from build123d import *

# Parameters (mm, degrees)
SKETCH1_W          = 190.5
SKETCH1_H          = 114.3
SKETCH1_R          = 2.413
SKETCH1_W_2        = 127
SKETCH1_H_2        = 82.55
BASE_FLANGE1_DEPTH = 2.38125
FILLET1_R          = 6.35
SKETCH2_W          = 36.53028
SKETCH2_H          = 15.875
CUT_EXTRUDE1_DEPTH = 2.54
FILLET2_R          = 6.35


# Sheet-metal steps are written as plain solids
with BuildPart() as part:
    # Sketch1 → Base-Flange1 (new body)
    with BuildSketch(Plane(origin=(0, 0, 0), x_dir=(1, 0, 0), z_dir=(0, 1, 0))):
        Rectangle(SKETCH1_W, SKETCH1_H)
        with Locations(Location((-76.2, -51.59375, 0), (0, 0, 270))):
            Circle(SKETCH1_R, mode=Mode.SUBTRACT)
        with Locations(Location((-50.8, -51.59375, 0), (0, 0, 270))):
            Circle(SKETCH1_R, mode=Mode.SUBTRACT)
        with Locations(Location((-25.4, -51.59375, 0), (0, 0, 270))):
            Circle(SKETCH1_R, mode=Mode.SUBTRACT)
        with Locations(Location((0, -51.59375, 0), (0, 0, 270))):
            Circle(SKETCH1_R, mode=Mode.SUBTRACT)
        with Locations(Location((25.4, -51.59375, 0), (0, 0, 270))):
            Circle(SKETCH1_R, mode=Mode.SUBTRACT)
        with Locations(Location((50.8, -51.59375, 0), (0, 0, 270))):
            Circle(SKETCH1_R, mode=Mode.SUBTRACT)
        with Locations(Location((76.2, -51.59375, 0), (0, 0, 270))):
            Circle(SKETCH1_R, mode=Mode.SUBTRACT)
        with Locations(Location((76.2, 51.59375, 0), (0, 0, 270))):
            Circle(SKETCH1_R, mode=Mode.SUBTRACT)
        with Locations(Location((50.8, 51.59375, 0), (0, 0, 270))):
            Circle(SKETCH1_R, mode=Mode.SUBTRACT)
        with Locations(Location((25.4, 51.59375, 0), (0, 0, 270))):
            Circle(SKETCH1_R, mode=Mode.SUBTRACT)
        with Locations(Location((0, 51.59375, 0), (0, 0, 270))):
            Circle(SKETCH1_R, mode=Mode.SUBTRACT)
        with Locations(Location((-25.4, 51.59375, 0), (0, 0, 270))):
            Circle(SKETCH1_R, mode=Mode.SUBTRACT)
        with Locations(Location((-50.8, 51.59375, 0), (0, 0, 270))):
            Circle(SKETCH1_R, mode=Mode.SUBTRACT)
        with Locations(Location((-76.2, 51.59375, 0), (0, 0, 270))):
            Circle(SKETCH1_R, mode=Mode.SUBTRACT)
        Rectangle(SKETCH1_W_2, SKETCH1_H_2, mode=Mode.SUBTRACT)
    extrude(amount=-BASE_FLANGE1_DEPTH)

    # Fillet1
    fillet1_edges = [part.edges().sort_by_distance(p)[0] for p in [
        (-95.25, -1.190625, -57.15),
        (95.25, -1.190625, -57.15),
        (95.25, -1.190625, 57.15),
        (-95.25, -1.190625, 57.15),
    ]]
    fillet(fillet1_edges, radius=FILLET1_R)

    # Sketch2 → Cut-Extrude1 (cut)
    with BuildSketch(Plane(origin=(0, 0, 0), x_dir=(1, 0, 0), z_dir=(0, 1, 0))):
        with Locations((40.94988, 49.2125)):
            Rectangle(SKETCH2_W, SKETCH2_H)
    extrude(amount=-CUT_EXTRUDE1_DEPTH, mode=Mode.SUBTRACT)

    # Fillet2
    # the kernel refuses this fillet: 6.35 mm, written as the material it takes off along each edge
    with BuildSketch(Plane(origin=(59.21502, 15.012118521, -41.275), x_dir=(0, 0, -1), z_dir=(0, -1, 0))) as fillet2_piece_1:
        with BuildLine():
            CenterArc((6.004847409, 6.35), FILLET2_R, 198.977692365, 71.022307635)
            Line((0, 4.28498), (-0.120096948, 4.2436796))
            ThreePointArc((-0.120096948, 4.2436796), (-0.127, 2.14249), (-0.127, 0))
            Line((-0.127, 0), (0, -0.127))
            Line((0, -0.127), (6.004847409, -0.127))
            Line((6.004847409, -0.127), (6.004847409, 0))
        make_face()
    extrude(amount=32.405487043, mode=Mode.SUBTRACT)
    with BuildSketch(Plane(origin=(22.68474, 15.875, -41.275), x_dir=(-1, 0, 0), z_dir=(0, -1, 0)), Plane(origin=(22.68474, 15.875, -57.15), x_dir=(0, 0, 1), z_dir=(0, -1, 0)), Plane(origin=(59.21502, 15.875, -57.15), x_dir=(1, 0, 0), z_dir=(0, -1, 0))) as fillet2_piece_2:
        with BuildLine():
            CenterArc((FILLET2_R, FILLET2_R), FILLET2_R, 180, 90)
            Line((0, FILLET2_R), (-FILLET2_R * 0.02, FILLET2_R))
            Line((-FILLET2_R * 0.02, FILLET2_R), (-FILLET2_R * 0.02, -FILLET2_R * 0.02))
            Line((-FILLET2_R * 0.02, -FILLET2_R * 0.02), (FILLET2_R, -FILLET2_R * 0.02))
            Line((FILLET2_R, -FILLET2_R * 0.02), (FILLET2_R, 0))
        make_face()
    extrude(amount=34.13125, mode=Mode.SUBTRACT)


solid = part.part
Could you check a few things on this model? Use its own coordinates, in mm. A direction names the side the tool comes from. Give positions to 0.01 mm unless a question says otherwise; leave off trailing zeros. Order: outer loops, then holes, each group sorted by start corner. A loop starts at its lowest first (then second) coordinate and runs counter-clockwise, first axis right, second up. Notation, with made-up numbers: (27.25, -13) - (86.25, -13) arc R15 cw to (86.25, 8) - close; hole circle Ø4 at (54.25, 49). An arc over 180 degrees is marked (long way). One line per item, written item: value. Start each with the question number.
1. Imagine slicing it at C-C on z = 30.5. List the corners of the cut face in (x, y) for me, plus the area to 3 significant figures.
2. Thinking about a two-plate mould opening in Z: for faces 1 (the face through (0.72, -1.17, -49.29)), 2 (the face through (-23, -2.381, 50)), 3 (the face through (93.34, -1.21, 55.34)), which applies, +Z half, -Z half, draft (parallel to the pull), parting line (faces both ways), or undercut?
3. If I drill on probe 1 along X at (y, z) = (-0.3, -23); probe 2 along Z at (x, y) = (5, -1.4) (3 decimals); probe 3 along Z at (x, y) = (65, -1.65), over which ranges is the centre line in solid material (lowest first)?
4. Imagine slicing it at B-B on x = -76.2. List the corners of the cut face in (y, z) for me.
5. Imagine slicing it at A-A on x = -36.5. List the corners of the cut face in (y, z) for me (3 decimals).
6. Imagine slicing it at D-D on y = -1.95. Give the number of separate pieces and of enclosed holes in the cut face, plus the area to 3 significant figures.
7. For P1, Ø4.5, axis at x = 0, z = -51.59, coming from the +Y side, with a flat end and sliding along its axis, tell me the tip position at first contact or that it passes through.
8. For faces 4 (the face through (-93.44, -1.21, 55.24)), 5 (the face through (20.775, -1.174, -55.339)), 6 (the face through (20.87, -1.17, -43.18)), which set-ups out of +Z, -Z, +X, -X, +Y, -Y let a thin tool reach every point of the face, with its end or its side?
Values:
1. outline: (-95.25, -2.38) - (-63.5, -2.38) - (-63.5, 0) - (-95.25, 0) - close; (63.5, -2.38) - (95.25, -2.38) - (95.25, 0) - (63.5, 0) - close
1. area: 151 mm²
2. face 1: undercut
2. face 2: draft
2. face 3: +Z half
3. probe 1: -95.25 to -63.5, 63.5 to 95.25
3. probe 2: -57.15 to -41.275, 41.275 to 57.15
3. probe 3: -57.12 to 57.15
4. outline: (-2.38, -57.15) - (0, -57.15) - (0, -54.01) - (-2.38, -54.01) - close; (-2.38, -49.18) - (0, -49.18) - (0, 49.18) - (-2.38, 49.18) - close; (-2.38, 54.01) - (0, 54.01) - (0, 57.15) - (-2.38, 57.15) - close
5. outline: (-2.381, -57.15) - (0, -57.15) - (0, -41.275) - (-2.381, -41.275) - close; (-2.381, 41.275) - (0, 41.275) - (0, 57.15) - (-2.381, 57.15) - close
6. separate pieces: 1
6. enclosed holes: 12
6. area: 10,400 mm²
7. P1: through
8. face 4: +Z, -X, +Y, -Y
8. face 5: -Z, +Y, -Y
8. face 6: +Y, -Y
